Autodesk Inventor part; units mm, degrees
ref_plane "YZ Plane" through (0, 0, 0) normal (1, 0, 0) x (0, 1, 0)
ref_plane "XZ Plane" through (0, 0, 0) normal (0, 1, 0) x (-1, 0, 0)
ref_plane "XY Plane" through (0, 0, 0) normal (0, 0, 1) x (1, 0, 0)
sketch "Sketch1" plane through (0, 0, 0) normal (1, 0, 0) x (0, 1, 0)
  point P0 (0, 0)
sketch "Sketch2" plane through (0, 0, 0) normal (1, 0, 0) x (0, 1, 0)
  arc A0 (10, 0) -> (-10, 0) centre (0, 0) ccw
  circle A1 centre (0, 0) radius 1.5
  line L0 (10, 0) -> (-10, 0)
  line L1 (-10, 0) -> (-10, -16)
  line L2 (0, -26) -> (10, -26)
  line L3 (10, -26) -> (10, 0)
  line L4 (0, -26) -> (0, -16)
  line L5 (0, -16) -> (-10, -16)
  dimension "d1" = 3
extrude "Extrusion1" add sketch "Sketch2" along normal blind 20
sketch "Sketch3" plane through (0, 10, 0) normal (0, 1, 0) x (1, 0, 0)
  line L0 (0, 26) -> (20, 26)
  line L1 (0, 16) -> (20, 16)
  arc A0 (20, 16) -> (0, 16) centre (10, 16) ccw
  line L2 (21.9475, 16) -> (-2.9161, 16)
  line L3 (-2.9161, 16) -> (-2.9161, 27.442)
  line L4 (-2.9161, 27.442) -> (21.9475, 27.442)
  line L5 (21.9475, 27.442) -> (21.9475, 16)
  point P0 (0, 0)
extrude "Extrusion2" cut sketch "Sketch3" against normal blind 20 contours L2 L3 L4 L5 A0
sketch "Sketch5" plane through (0, 10, 0) normal (0, 1, 0) x (1, 0, 0)
  line L0 (0, -10) -> (20, -10)
  line L1 (0, -10) -> (4.9, -10)
  line L2 (4.9, -10) -> (4.9, 10)
  line L3 (4.9, 10) -> (17, 10)
  line L4 (17, 10) -> (17, -10)
  line L5 (17, -10) -> (4.9, -10)
  point P0 (0, 0)
  dimension "d10" = 4.9
  dimension "d11" = 20
  dimension "d12" = 12.1
extrude "Extrusion3" cut sketch "Sketch5" against normal blind 20
sketch "Sketch6" plane through (0, 0, 0) normal (-1, 0, 0) x (0, 0, 1)
  arc A0 (0, 2.5) -> (0, -2.5) centre (0, 0) ccw
  line L0 (0, 2.5) -> (12.401, 2.5)
  line L1 (12.401, 2.5) -> (12.401, -2.5)
  line L2 (12.401, -2.5) -> (0, -2.5)
  dimension "d15" = 5
extrude "Extrusion4" cut sketch "Sketch6" against normal blind 5
sketch "Sketch7" plane through (0, 0, 0) normal (-1, 0, 0) x (0, 0, 1)
  line L0 (-16, -10) -> (12.5782, -10)
  line L1 (12.5782, -10) -> (12.5782, -5)
  line L2 (12.5782, -5) -> (-16, -5)
  line L3 (-16, -5) -> (-16, -10)
  point P0 (0, 0)
  dimension "d18" = 5
extrude "Extrusion5" cut sketch "Sketch7" against normal through all
sketch "Sketch8" plane through (0, 10, 0) normal (0, 1, 0) x (1, 0, 0)
  line L0 (0, 16) -> (20, 16)
  circle A0 centre (10, 16) radius 2
  point P0 (0, 0)
  dimension "d21" = 4
extrude "Extrusion6" cut sketch "Sketch8" against normal through all
sketch "Sketch9" plane through (0, -5, -16) normal (0, -1, 0) x (1, 0, 0)
  line L0 (0, 0) -> (8, 0)
  line L1 (12, 0) -> (20, 0)
  line L2 (8, 0) -> (12, 0)
  circle A0 centre (10, 0) radius 4.5
  point P0 (0, 16)
  dimension "d24" = 9
extrude "Extrusion7" cut sketch "Sketch9" against normal blind 10
sketch "Sketch12" plane through (0, -5, -16) normal (0, -1, 0) x (1, 0, 0)
  arc A0 (14.5, 0) -> (5.5, 0) centre (10, 0) ccw
  line L0 (4.9, 6) -> (17, 6)
  line L1 (9, 6) -> (9, 4.2062)
  line L2 (11, 6) -> (11, 4.2062)
  line L3 (9, 4.2062) -> (11, 4.2062)
  line L4 (9, 6) -> (11, 6)
  point P0 (0, 16)
extrude "Extrusion8" cut sketch "Sketch12" against normal blind 4
sketch "Sketch13" plane through (0, -5, -16) normal (0, -1, 0) x (1, 0, 0)
  arc A0 (5.5, 0) -> (-5.5, 0) centre (0, 0) ccw
  arc A1 (25.5, 0) -> (14.5, 0) centre (20, 0) ccw
  line L0 (26.0588, 0) -> (26.0588, -15.4765)
  line L1 (26.0588, -15.4765) -> (-5.5, -15.4765)
  line L2 (-5.5, -15.4765) -> (-5.5, 0)
  line L3 (5.5, 0) -> (14.5, 0)
  line L4 (25.5, 0) -> (26.0588, 0)
  point P0 (0, 16)
  dimension "d33" = 11
  dimension "d34" = 11
extrude "Extrusion9" cut sketch "Sketch13" against normal blind 5
sketch "Sketch14" plane through (20, 0, 0) normal (1, 0, 0) x (0, 0, -1)
  circle A0 centre (3.94, 7.53) radius 1.5
  point P0 (0, 0)
  point P1 (0, 10)
  dimension "d39" = 3
extrude "Extrusion10" cut sketch "Sketch14" against normal blind 5
sketch "Sketch15" plane through (20, 0, 0) normal (1, 0, 0) x (0, 0, -1)
  circle A0 centre (0, 0) radius 1.5
  dimension "d43" = 3
extrude "Extrusion11" cut sketch "Sketch15" against normal blind 5
sketch "Sketch16" plane through (4.9, 10, 0) normal (1, 0, 0) x (0, 0, -1)
  line L0 (0, 0) -> (-1.5, 0)
  line L1 (-1.5, 0) -> (-1.5, -1.5)
  line L2 (-1.5, -1.5) -> (11.5, -1.5)
  line L3 (11.5, -1.5) -> (11.5, 0)
  line L4 (16, 0) -> (0, 0)
  line L5 (11.5, 0) -> (0, 0)
  point P0 (0, -10)
  dimension "d46" = 1.5
  dimension "d47" = 1.5
  dimension "d48" = 13
extrude "Extrusion12" add sketch "Sketch16" along normal blind 7
sketch "Sketch17" plane through (0, 0, 0) normal (-1, 0, 0) x (0, 0, 1)
  line L0 (9.6825, 2.5) -> (0, 2.5)
  line L1 (0, 2.5) -> (7, 2.5)
  line L2 (7, 2.5) -> (7, 10)
  line L3 (7, 10) -> (0, 10)
  line L4 (0, 10) -> (0, 2.5)
  point P0 (0, 0)
  dimension "d51" = 7
  dimension "d52" = 7.5
extrude "Extrusion13" add sketch "Sketch17" against normal blind 4.9
sketch "Sketch18" plane through (10, 10, -16) normal (0, 1, 0) x (1, 0, 0)
  circle A0 centre (-7.55, -20) radius 0.5
  line L0 (-5.1, -23) -> (-10, -23)
  line L1 (-7.55, -23) -> (-7.55, -20)
  point P0 (-10, -16)
  dimension "d55" = 1
  dimension "d58" = 3
extrude "Extrusion14" cut sketch "Sketch18" against normal up to next
sketch "Sketch19" plane through (17, -5, -10) normal (0, 0, 1) x (1, 0, 0)
  line L0 (-5.1, 13.5) -> (-12.1, 13.5)
  line L1 (-5.1, 13.5) -> (-5.1, 8.65)
  line L2 (-5.1, 8.65) -> (-7.1, 8.65)
  line L3 (-7.1, 8.65) -> (-7.1, 13.5)
  line L4 (-5.1, 15) -> (-5.1, 13.5)
  line L5 (-7.1, 13.5) -> (-5.1, 13.5)
  point P0 (-17, 5)
  dimension "d59" = 4.85
  dimension "d60" = 2
extrude "Extrusion15" add sketch "Sketch19" along normal blind 12
sketch "Sketch20" plane through (11.9, 10, 0) normal (1, 0, 0) x (0, 0, -1)
  circle A0 centre (3.94, -2.47) radius 1.5
  circle A1 centre (3.94, -2.47) radius 1.5
  point P0 (0, -10)
extrude "Extrusion16" cut sketch "Sketch20" against normal blind 2
sketch "Sketch21" plane through (11.9, 10, 0) normal (1, 0, 0) x (0, 0, -1)
  line L0 (-7.3238, -1.5) -> (-7.3238, -7.2177)
  line L1 (-7.3238, -7.2177) -> (-1.5, -7.2177)
  line L2 (-1.5, -7.2177) -> (4.1962, -7.2177)
  line L3 (10, -6.35) -> (-2, -6.35)
  line L4 (-1.5, 0) -> (-1.5, -1.5)
  line L5 (-1.5, 0) -> (-7.3238, 0)
  line L6 (-7.3238, 0) -> (-7.3238, -1.5)
  line L7 (-1.5, -0.1522) -> (-1.5, 0)
  line L8 (4.1962, -7.2177) -> (6.1782, -7.2177)
  line L9 (6.1782, -7.2177) -> (6.1782, -6.35)
  arc A0 (-1.5, 0) -> (6.141, -6.35) centre (6.8954, 2.33) ccw
  point P0 (0, -10)
  point P1 (4.1962, -6.35)
  point P2 (3.0513, -6.35)
extrude "Extrusion17" cut sketch "Sketch21" against normal blind 7
properties part number "knuckle"
Check sheet for the modelled part. Datum: model origin and axes. Units: mm. A direction names the side the tool comes from. Coordinates: 2 decimals unless noted, no trailing zeros. Loops run counter-clockwise (first coordinate to the right, second up) from the corner with the lowest first, then second, coordinate; pieces in that order, holes last. Notation, with made-up numbers: M 74,76.25 L 86,76.25 A16 cw 86,87.25 Z; hole C 33.5,-13 d7. An arc over 180 degrees is marked long. Answer as a JSON object with one key per item and string values.
1. Sectioned sample at D-D on y = 7.53. Record the cut outline in (x, z), and give its area (3 significant figures).
Outcome:
{"outline": "M 0,-16 A10 ccw 20,-16 L 20,-5.44 L 17,-5.44 L 17,-10 L 11.9,-10 L 11.9,-5.44 L 9.9,-5.44 L 9.9,-10 L 4.9,-10 L 4.9,7 L 0,7 Z; M 9.9,-2.44 L 11.9,-2.44 L 11.9,0.38 L 9.9,0.38 Z; M 17,-2.44 L 20,-2.44 L 20,6.58 L 17,6.58 Z; hole C 2.45,4 d1; hole C 10,-16 d4", "area": "403 mm²"}
2. Sectioned sample at C-C on y = -0.5. Record the cut outline in (x, z), and give its area (3 significant figures).
Outcome:
{"outline": "M 0,-10.5 A5.5 cw 5.5,-16 A4.5 cw 14.5,-16 A5.5 cw 20,-10.5 L 20,-1.41 L 17,-1.41 L 17,-10 L 4.9,-10 L 4.9,-2.45 L 0,-2.45 Z; M 17,1.41 L 20,1.41 L 20,9.99 L 17,9.99 Z", "area": "129 mm²"}
3. Depth check by flat-ended pin: P1, Ø4.5, axis at x = 10, z = -16, coming from the -Y side; P2, Ø4.5, axis at x = 7.5, z = -19.5, coming from the -Y side; P3, Ø1.6, axis at x = 11, z = -7.5, coming from the -Y side. Enter the tip coordinate at first touch or a pass-through.
Outcome:
{"P1": "y = 5", "P2": "y = 0", "P3": "y = 3.65"}
4. Sectioned sample at B-B on x = 11.5. Record the cut outline in (y, z).
Outcome:
{"outline": "M -5,-11.76 L 5,-11.76 L 5,-14.68 L 10,-14.68 L 10,1.5 A8.71 ccw 3.65,-6.14 L 3.65,-10 L -5,-10 Z; M 0,-25.89 L 10,-25.89 L 10,-17.32 L 5,-17.32 L 5,-20.24 L 0,-20.24 Z; hole C 7.53,-3.94 d3"}
5. Access from +Z, -Z, +X, -X, +Y, -Y to the whole of each face (thin tool, end or side, straight path). Record for faces 1 (the flat face through (17, 3, 0)), 2 (the cylindrical face through (18.521, 8.795, -4.746)), 3 (the cylindrical face through (18.479, 4.873, 8.733)).
Outcome:
{"face 1": "+Z, +Y, -Y", "face 2": "+X", "face 3": "+Z, +X"}
6. Sectioned sample at A-A on z = 2.5. Record the cut outline in (x, y), and give its area (3 significant figures).
Outcome:
{"outline": "M 0,-5 L 4.9,-5 L 4.9,-2.5 L 0,-2.5 Z; M 0,2.5 L 4.9,2.5 L 4.9,10 L 0,10 Z; M 17,-5 L 20,-5 L 20,9.68 L 17,9.68 Z", "area": "93.0 mm²"}
7. Scan lines: L1, parallel to X at y = 6.3, z = -16; L2, parallel to X at y = -2.5, z = -9; L3, parallel to X at y = 8, z = 4. Record each from-to range of solid material in increasing order. Write a range as from..to.
Outcome:
{"L1": "0..8, 12..20", "L2": "0..4.9, 17..20", "L3": "0..1.95, 2.95..4.9, 17..20"}
8. Release check for a two-part mould opening along Z. For faces 4 (the cylindrical face through (2.4, 0.1, -2.5)), 5 (the cylindrical face through (10, 8, -18)), 6 (the flat face through (3, -5, -3)), 7 (the cylindrical face through (10.914, 8.795, -4.746)) record: pulls with the +Z half, pulls with the -Z half, needs draft (parallel to the pull), parting line crosses it, or undercut.
Outcome:
{"face 4": "pulls with the +Z half", "face 5": "undercut", "face 6": "needs draft", "face 7": "undercut"}
